Part model, mm, in its own coordinate system. A direction names the side the tool comes from. Give positions to 0.01 mm unless a question says otherwise; leave off trailing zeros. Order: outer loops, then holes, each group sorted by start corner. A loop starts at its lowest first (then second) coordinate and runs counter-clockwise, first axis right, second up. Notation, with made-up numbers: (66, 50) - (106, 50) arc R19 ccw to (106, 76) - close; hole circle Ø9 at (16, -9). An arc over 180 degrees is marked (long way). One line per item, written item: value.
```python
from build123d import *
from OCP.BRepFilletAPI import BRepFilletAPI_MakeFillet
from build123d.topology import SkipClean

# Parameters (mm, degrees)
BOSS_EXTRUDE1_DEPTH = 6
FILLET1_R           = 6
FILLET2_R1          = 10
FILLET2_R2          = 15
CUT_EXTRUDE1_DEPTH  = 17.5
SKETCH5_R           = 4
BOSS_EXTRUDE2_DEPTH = 6
CUT_EXTRUDE2_DEPTH  = 6
SKETCH7_R           = 2.7
CUT_EXTRUDE4_DEPTH  = 96.469302576


with BuildPart() as part:
    # Sketch1 → Boss-Extrude1 (new, symmetric)
    with BuildSketch(Plane(origin=(0, 0, 0), x_dir=(1, 0, 0), z_dir=(0, 1, 0))):
        Polygon((50, 37.5), (50, 22.5), (-50, 22.5), (-50, -22.5), (50, -22.5), (50, -37.5), (-65, -37.5), (-65, 37.5), align=None)
    extrude(amount=BOSS_EXTRUDE1_DEPTH, both=True)

    # Fillet1
    fillet1_edges = [part.edges().sort_by_distance(p)[0] for p in [
        (50, 6, -30),
        (50, -6, -30),
        (50, -6, 30),
        (50, 6, 30),
    ]]
    fillet(fillet1_edges, radius=FILLET1_R - 0.0001)  # a hair under: the kernel refuses the full size

    # Fillet2: one fillet with a radius per group of edges: ONE call of the kernel's fillet builder (fillet() takes one radius for all edges)
    fillet2_edges_1 = [part.edges().sort_by_distance(p)[0] for p in [
        (-50, 0, 22.5),
        (-50, 0, -22.5),
    ]]
    fillet2_edges_2 = [part.edges().sort_by_distance(p)[0] for p in [
        (-65, 0, 37.5),
        (-65, 0, -37.5),
    ]]
    fillet2 = BRepFilletAPI_MakeFillet(part.part.solid().wrapped)
    for e in fillet2_edges_1:
        fillet2.Add(FILLET2_R1, e.wrapped)
    for e in fillet2_edges_2:
        fillet2.Add(FILLET2_R2, e.wrapped)
    add(Compound.cast(fillet2.Shape()), mode=Mode.REPLACE)

    # Sketch4 → Cut-Extrude1 (cut, symmetric)
    with BuildSketch(Plane.XY):
        Polygon((-63, 6), (-51, 2.784609691), (-51, 6), align=None)
    extrude(amount=CUT_EXTRUDE1_DEPTH, both=True, mode=Mode.SUBTRACT)

    # Sketch5 → Boss-Extrude2 (add)
    with BuildSketch(Plane(origin=(-2.720199781, -10.151923789, 0), x_dir=(0.9659258262890701, -0.25881904510251424, 0), z_dir=(0.25881904510251424, 0.9659258262890701, 0))):
        with Locations((-56.610686369, 10)):
            Circle(SKETCH5_R)
        with Locations((-56.610686369, -10)):
            Circle(SKETCH5_R)
    extrude(amount=BOSS_EXTRUDE2_DEPTH)

    # Sketch6 → Cut-Extrude2 (cut)
    with BuildSketch(Plane.XY.offset(37.5)):
        with BuildLine():
            Line((42.25, -2.056088519), (42.25, 2.056088519))
            ThreePointArc((42.25, 2.056088519), (44, 2.7), (45.75, 2.056088519))
            Line((45.75, 2.056088519), (45.75, -2.056088519))
            ThreePointArc((45.75, -2.056088519), (44, -2.7), (42.25, -2.056088519))
        make_face()
    extrude(amount=-CUT_EXTRUDE2_DEPTH, mode=Mode.SUBTRACT)

    # Sketch7 → Cut-Extrude4 (cut, through all)
    with SkipClean():  # the faces are left unmerged after this step: merging them gives an invalid solid
        with BuildSketch(Plane.XY.offset(31.5)):
            with Locations((44, 0)):
                Circle(SKETCH7_R)
        extrude(amount=-CUT_EXTRUDE4_DEPTH, mode=Mode.SUBTRACT)


solid = part.part
```
1) Cut at C-C, the plane x = -45. Give the cut face in (y, z).
Outcome:
outline: (-6, -37.5) - (6, -37.5) - (6, -21.16) - (-6, -21.16) - close; (-6, 21.16) - (6, 21.16) - (6, 37.5) - (-6, 37.5) - close
2) Pin check, flat tips, straight feed: pin 1 (6 mm diameter, centred on x = -52.5, y = 5.5, fed in from +Z); pin 2 (1 mm diameter, centred on x = -7, z = -26, fed in from +Y); pin 3 (4.5 mm diameter, centred on y = 0, z = 34.5, fed in from -X); pin 4 (6 mm diameter, centred on y = -2.5, z = -12, fed in from +X). Stop position of each tip, or through.
Outcome:
pin 1: stops at z = 37.5
pin 2: stops at y = 6
pin 3: stops at x = -61.4
pin 4: stops at x = -49.68
3) Cut at A-A, the plane x = 2. Give the cut face in (y, z), then the cut area to 3 significant figures.
Outcome:
outline: (-6, -37.5) - (6, -37.5) - (6, -22.5) - (-6, -22.5) - close; (-6, 22.5) - (6, 22.5) - (6, 37.5) - (-6, 37.5) - close
area: 360 mm^2
4) Drill centre lines: line 1 along Z through (x, y) = (-31.5, -0.75); line 2 along Y through (x, z) = (44, 27.75); line 3 along Y through (x, z) = (-26.5, -25.5). Where is each one in solid material? Low to high. Write a range as from..to.
Outcome:
line 1: z = -37.5..-22.5, 22.5..37.5
line 2: y = -6..-2.7, 2.7..6
line 3: y = -6..6
5) Which spindle directions (+Z, -Z, +X, -X, +Y, -Y) get a long thin tool onto all of the face, cutting with end or side? Do faces 4 (the flat face through (4, 0, 22.5)), 5 (the flat face through (45.75, 0, 35)), 6 (the cylindrical face through (46.575, 0.811, -29.895)), 7 (the flat face through (-54, 5, -17.5)), 8 (the flat face through (1, 0, 37.5)). Say none if no direction does.
Outcome:
face 4: +X, +Y, -Y
face 5: +Z, -Z
face 6: -Z
face 7: +Y
face 8: +Z, +X, -X, +Y, -Y
6) Mould opens along Z. For faces 1 (the flat face through (-54, 5, 17.5)), 2 (the flat face through (-10, 6, -26)), 3 (the cylindrical face through (-60.49, 0.08, -33.22)) say: released by +Z, released by -Z, zero draft, split by the parting line, or undercut.
Outcome:
face 1: undercut
face 2: zero draft
face 3: released by -Z
